from build123d import *

# Parameters (mm, degrees)
EXTRUDE_1_DEPTH = 4.3
FILLET_1_R      = 3
SHELL_1_T       = -2
SKETCH_3_R      = 3.45
SKETCH_3_R_2    = 2.95
EXTRUDE_2_DEPTH = 10


with BuildPart() as part:
    # 草图1 → 凸台-拉伸1 (new body)
    with BuildSketch(Plane.XY):
        with BuildLine():
            Line((3, 0), (37, 0))
            ThreePointArc((37, 0), (39.121320344, 0.878679656), (40, 3))
            Line((40, 3), (40, 77))
            ThreePointArc((40, 77), (39.121320344, 79.121320344), (37, 80))
            Line((37, 80), (3, 80))
            ThreePointArc((3, 80), (0.878679656, 79.121320344), (0, 77))
            Line((0, 77), (0, 3))
            ThreePointArc((0, 3), (0.878679656, 0.878679656), (3, 0))
        make_face()
    extrude(amount=EXTRUDE_1_DEPTH)

    # 圆角1
    fillet_1_edges = [part.edges().sort_by_distance(p)[0] for p in [
        (20, 0, 0),
        (0.878679656, 0.878679656, 0),
        (0, 40, 0),
        (0.878679656, 79.121320344, 0),
        (20, 80, 0),
        (39.121320344, 79.121320344, 0),
        (40, 40, 0),
        (39.121320344, 0.878679656, 0),
    ]]
    fillet(fillet_1_edges, radius=FILLET_1_R)

    # 抽壳1
    shell_1_openings = [part.faces().sort_by_distance(p)[0] for p in [
        (20, 40, 4.3),
    ]]
    offset(amount=SHELL_1_T, openings=shell_1_openings, kind=Kind.INTERSECTION)

    # 草图3 → 凸台-拉伸2 (add)
    # profile 1 of 2: a face of its own
    with BuildSketch(Plane.XY.offset(2)):
        with Locations((20, 20)):
            Circle(SKETCH_3_R)
        with Locations((20, 20)):
            Circle(SKETCH_3_R_2, mode=Mode.SUBTRACT)
    # profile 2 of 2: a face of its own
    with BuildSketch(Plane.XY.offset(2)):
        with Locations(Location((20, 60, 0), (0, 0, 180))):
            Circle(SKETCH_3_R)
        with Locations(Location((20, 60, 0), (0, 0, 180))):
            Circle(SKETCH_3_R_2, mode=Mode.SUBTRACT)
    extrude(amount=EXTRUDE_2_DEPTH)


solid = part.part
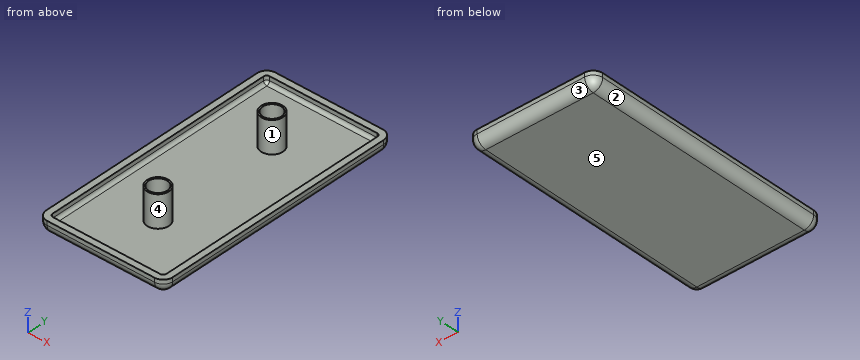
Part model, mm, in its own coordinate system. Face numbers are marked on the shaded views. A direction names the side the tool comes from. Give positions to 0.01 mm unless a question says otherwise; leave off trailing zeros. Loops run counter-clockwise (first coordinate to the right, second up) from the corner with the lowest first, then second, coordinate; pieces in that order, holes last.
(1) Band-saw the part on D-D (z = 1.25). Write the cut outline in (x, y).
Return value:
outline: (0.56, 3) arc R2.44 ccw to (3, 0.56) - (37, 0.56) arc R2.44 ccw to (39.44, 3) - (39.44, 77) arc R2.44 ccw to (37, 79.44) - (3, 79.44) arc R2.44 ccw to (0.56, 77) - close
(2) Pull direction Y, two halves, no side cores. Call the marked faces 3, 4 and 5: pulls with the +Y half, pulls with the -Y half, needs draft (parallel to the pull), parting line crosses it, or undercut.
Return value:
face 3: pulls with the +Y half
face 4: undercut
face 5: needs draft
(3) Band-saw the part on C-C (x = 8.5). Write the cut outline in (y, z), and give its area (3 significant figures).
Return value:
outline: (0, 3) arc R3 ccw to (3, 0) - (77, 0) arc R3 ccw to (80, 3) - (80, 4.3) - (78, 4.3) - (78, 3) arc R1 cw to (77, 2) - (3, 2) arc R1 cw to (2, 3) - (2, 4.3) - (0, 4.3) - close
area: 166 mm2
(4) Band-saw the part on A-A (y = 20). Write the cut outline in (x, z), and give its area (3 significant figures).
Return value:
outline: (0, 3) arc R3 ccw to (3, 0) - (37, 0) arc R3 ccw to (40, 3) - (40, 4.3) - (38, 4.3) - (38, 3) arc R1 cw to (37, 2) - (23.45, 2) - (23.45, 12) - (22.95, 12) - (22.95, 2) - (17.05, 2) - (17.05, 12) - (16.55, 12) - (16.55, 2) - (3, 2) arc R1 cw to (2, 3) - (2, 4.3) - (0, 4.3) - close
area: 95.8 mm2
(5) Pin check, flat tips, straight feed: pin 1 (3 mm diameter, centred on x = 15.5, z = 6, fed in from +Y); pin 2 (4.5 mm diameter, centred on x = 19.5, y = 20, fed in from +Z); pin 3 (1 mm diameter, centred on x = 13.5, z = 6.5, fed in from -Y); pin 4 (6 mm diameter, centred on x = 18, z = 10, fed in from +Y). Stop position of each tip, or through.
Return value:
pin 1: stops at y = 61.7
pin 2: stops at z = 2
pin 3: passes through
pin 4: stops at y = 63.45
(6) Drill centre lines: line 1 along Y through (x, z) = (20, 7.25); line 2 along X through (y, z) = (60, 8.25); line 3 along Z through (x, y) = (27.5, 36.5). Where is each one in solid material? Low to high.
Return value:
line 1: y = 16.55 to 17.05, 22.95 to 23.45, 56.55 to 57.05, 62.95 to 63.45
line 2: x = 16.55 to 17.05, 22.95 to 23.45
line 3: z = 0 to 2
(7) Band-saw the part on B-B (z = 8). Write the cut outline in (x, y), and give its area (3 significant figures).
Return value:
outline: circle Ø6.9 at (20, 20); circle Ø6.9 at (20, 60); hole circle Ø5.9 at (20, 20); hole circle Ø5.9 at (20, 60)
area: 20.1 mm2
(8) 3-axis set-ups, long thin cutter, end or side, ignore diameter. For the marked faces 1 and 2: which of +Z, -Z, +X, -X, +Y, -Y reach the whole face in a straight line?
Return value:
face 1: +Z
face 2: -Z, -X, +Y, -Y
